```python
from build123d import *

# Parameters (mm, degrees)
SKETCH1_W                       = 45
SKETCH1_H                       = 40
SKETCH1_R                       = 16
BOSS_EXTRUDE1_DEPTH             = 3.5
M3X0_5_TAPPED_HOLE2_D           = 2.5
M3X0_5_TAPPED_HOLE2_DEPTH       = 25
M3X0_5_TAPPED_HOLE2_TIP         = 0.751075774
CUT_EXTRUDE1_DEPTH              = 5
CBORE_FOR_M3_SBHCS1_D           = 3.4
CBORE_FOR_M3_SBHCS1_DEPTH       = 7
CBORE_FOR_M3_SBHCS1_CBORE_D     = 6.7
CBORE_FOR_M3_SBHCS1_CBORE_DEPTH = 2.65
CBORE_FOR_M3_SBHCS1_TIP         = 1.021463052
F_3D_PRINTING_TOLERANCE_BY      = 0.05


with BuildPart() as part:
    # Sketch1 → Boss-Extrude1 (new, symmetric)
    with BuildSketch(Plane.XY):
        Rectangle(SKETCH1_W, SKETCH1_H)
        with Locations((0, -2.5)):
            Circle(SKETCH1_R, mode=Mode.SUBTRACT)
    extrude(amount=BOSS_EXTRUDE1_DEPTH, both=True)

    # M3x0.5 Tapped Hole2
    with Locations(Plane(origin=(0, -25, 71.05), x_dir=(0, 0, 1), z_dir=(0, -1, 0))):
        with Locations((-41.05, -18.5), (-71.05, 18.5), (-71.05, -18.5), (-41.05, 18.5)):
            Hole(M3X0_5_TAPPED_HOLE2_D / 2, depth=M3X0_5_TAPPED_HOLE2_DEPTH)
            with Locations((0, 0, -(M3X0_5_TAPPED_HOLE2_DEPTH + M3X0_5_TAPPED_HOLE2_TIP / 2))):  # 118° drill point
                Cone(0, M3X0_5_TAPPED_HOLE2_D / 2, M3X0_5_TAPPED_HOLE2_TIP, mode=Mode.SUBTRACT)

    # Sketch7 → Cut-Extrude1 (cut, symmetric)
    with BuildSketch(Plane.XY):
        Polygon((10.5, -20), (16.5, -9), (22.5, -9), (22.5, -20), align=None)
        Polygon((-10.5, -20), (-16.5, -9), (-22.5, -9), (-22.5, -20), align=None)
    extrude(amount=CUT_EXTRUDE1_DEPTH, both=True, mode=Mode.SUBTRACT)

    # CBORE for M3 SBHCS1
    with Locations(Plane(origin=(0, -2.5, -3.5), x_dir=(-1, 0, 0), z_dir=(0, 0, -1))):
        with Locations((-18, 18)):
            CounterBoreHole(CBORE_FOR_M3_SBHCS1_D / 2, CBORE_FOR_M3_SBHCS1_CBORE_D / 2, CBORE_FOR_M3_SBHCS1_CBORE_DEPTH, depth=CBORE_FOR_M3_SBHCS1_DEPTH)
            with Locations((0, 0, -(CBORE_FOR_M3_SBHCS1_DEPTH + CBORE_FOR_M3_SBHCS1_TIP / 2))):  # 118° drill point
                Cone(0, CBORE_FOR_M3_SBHCS1_D / 2, CBORE_FOR_M3_SBHCS1_TIP, mode=Mode.SUBTRACT)

    # 3D printing tolerance: a curved face moved inward by 0.05
    add(Solid.thicken(part.faces().sort_by_distance((-16, -2.5, 0))[0], -F_3D_PRINTING_TOLERANCE_BY), mode=Mode.SUBTRACT)


solid = part.part
```
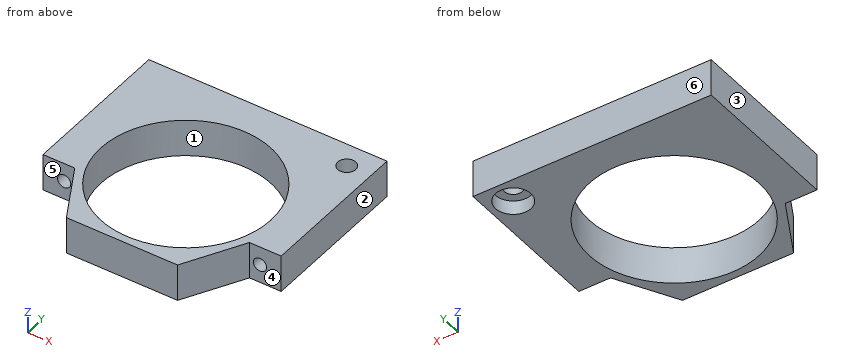
Input: part model. Units: mm. Frame: model coordinates. Face numbers are marked on the shaded views. A direction names the side the tool comes from. Round coordinates to 2 decimals unless told otherwise and drop trailing zeros. Loops run counter-clockwise (first coordinate to the right, second up) from the corner with the lowest first, then second, coordinate; pieces in that order, holes last. Notation, with made-up numbers: M 81,58.25 L 88,58.25 A19 ccw 88,89.25 Z; hole C 86.5,4.5 d8. An arc over 180 degrees is marked long. Answer in a Markdown table with one row per item. Add a question column.
1. Section B-B (x = 0). Output: boundary loops of the cut face in (y, z), and give its area (3 significant figures).
2. Section C-C (z = -1.75). Output: boundary loops of the cut face in (x, y), and give its area (3 significant figures).
3. Section A-A (y = -2.5). Output: boundary loops of the cut face in (x, z), and give its area (3 significant figures).
4. Section D-D (y = 9). Output: boundary loops of the cut face in (x, z), and give its area (3 significant figures).
5. Set-up query: the marked faces 5 and 6. Return all of +Z, -Z, +X, -X, +Y, -Y with unobstructed straight access to the full face (end or side cutting, diameter ignored); none if empty.
6. Ray query, probe 1 along Y at (x, z) = (18, 1.7); probe 2 along X at (y, z) = (-3, -2.5); probe 3 along X at (y, z) = (15.5, 2). Return the intervals inside material, ascending.
7. Contact query for flat-ended pins moving along their axis: pin 1 (2 mm diameter, centred on x = 18, y = 16.5, fed in from -Z); pin 2 (3 mm diameter, centred on x = 18.5, z = 0, fed in from -Y). Output: stop coordinate, or through.
8. Mould query, pull axis X, two halves, no side actions, for the marked faces 1, 2, 3 and 4. Classes: released by +X, released by -X, zero draft, split by the parting line, or undercut.
Values follow:
| question | item | result |
|---|---|---|
| 1 | outline | M -20,-3.5 L -18.55,-3.5 L -18.55,3.5 L -20,3.5 Z; M 13.55,-3.5 L 20,-3.5 L 20,3.5 L 13.55,3.5 Z |
| 1 | area | 55.3 mm^2 |
| 2 | outline | M -22.5,-9 L -16.5,-9 L -10.5,-20 L 10.5,-20 L 16.5,-9 L 22.5,-9 L 22.5,20 L -22.5,20 Z; hole C 0,-2.5 d32.1; hole C 18,15.5 d6.7 |
| 2 | area | 757 mm^2 |
| 3 | outline | M -22.5,-3.5 L -16.05,-3.5 L -16.05,3.5 L -22.5,3.5 Z; M 16.05,-3.5 L 22.5,-3.5 L 22.5,3.5 L 16.05,3.5 Z; hole C -18.5,0 d2.5; hole C 18.5,0 d2.5 |
| 3 | area | 80.5 mm^2 |
| 4 | outline | M -22.5,-3.5 L -11.2,-3.5 L -11.2,3.5 L -22.5,3.5 Z; M 11.2,-3.5 L 22.5,-3.5 L 22.5,3.5 L 11.2,3.5 Z |
| 4 | area | 158 mm^2 |
| 5 | face 5 | +Z, -Z, -X, -Y |
| 5 | face 6 | +Z, -Z, +X, -X, +Y |
| 6 | probe 1 | -9 to 13.8, 17.2 to 20 |
| 6 | probe 2 | -22.5 to -16.04, 16.04 to 22.5 |
| 6 | probe 3 | -22.5 to 16.3, 19.7 to 22.5 |
| 7 | pin 1 | z = -0.85 |
| 7 | pin 2 | y = -9 |
| 8 | face 1 | undercut |
| 8 | face 2 | released by +X |
| 8 | face 3 | released by -X |
| 8 | face 4 | zero draft |
